For this review, take the finished solid that the model builds, in its own axes (mm). A direction names the side the tool comes from. Give positions to 0.01 mm unless a question says otherwise; leave off trailing zeros. Write each loop counter-clockwise with the first axis right and the second up, starting at its lowest first coordinate (ties: lowest second). Pieces come first, ordered by that corner, then holes. Notation, with made-up numbers: (86, 33) -> (143, 33) arc R17 ccw to (143, 42) -> close; hole circle Ø2 at (74.5, -11). An arc over 180 degrees is marked (long way). Return JSON: item names as keys, results as strings.
from build123d import *

# Parameters (mm, degrees)
SKETCH1_W           = 8
SKETCH1_H           = 1.2
SKETCH1_W_2         = 1
SKETCH1_H_2         = 4.1
REVOLVE1_ANGLE      = 180
SKETCH2_W           = 6.21
SKETCH2_H           = 1.5
CUT_EXTRUDE1_DEPTH  = 14.787313009
CUT_EXTRUDE2_DEPTH  = 14.787313009
SKETCH4_W           = 3.4
SKETCH4_H           = 2
BOSS_EXTRUDE1_DEPTH = 1.2
SKETCH6_W           = 2.8
SKETCH6_H           = 5
BOSS_EXTRUDE3_DEPTH = 1.2
BOSS_EXTRUDE4_DEPTH = 0.6
SKETCH8_W           = 4.65
SKETCH8_H           = 2.2
SKETCH8_W_2         = 16.704991512
SKETCH8_H_2         = 4.40240097
CUT_EXTRUDE3_DEPTH  = 10
SKETCH5_W           = 3.2
SKETCH5_H           = 5.3
BOSS_EXTRUDE5_DEPTH = 2.5
SKETCH9_W           = 2
SKETCH9_H           = 3.6
CUT_EXTRUDE4_DEPTH  = 5
CHAMFER1_SIZE       = 1


with BuildPart() as part:
    # Sketch1 → Revolve1 (revolve)
    with BuildSketch(Plane.XY):
        with Locations((4, 4.7)):
            Rectangle(SKETCH1_W, SKETCH1_H)
        with Locations((8.5, 4.7)):
            Rectangle(SKETCH1_W_2, SKETCH1_H)
        with Locations((8.5, 2.05)):
            Rectangle(SKETCH1_W_2, SKETCH1_H_2)
    revolve(axis=Axis((0, 0, 0), (0, 1, 0)), revolution_arc=REVOLVE1_ANGLE)

    # Sketch2 → Cut-Extrude1 (cut, through all)
    with BuildSketch(Plane.XY):
        with Locations((0, 3.35)):
            Rectangle(SKETCH2_W, SKETCH2_H)
    extrude(amount=-CUT_EXTRUDE1_DEPTH, mode=Mode.SUBTRACT)

    # Sketch3 → Cut-Extrude2 (cut, through all)
    with BuildSketch(Plane(origin=(0, 5.3, 0), x_dir=(1, 0, 0), z_dir=(0, 1, 0))):
        Polygon((-2.2, 5.8), (-3.6, 5.8), (-3.6, 0), (3.6, 0), (3.6, 5.8), (2.2, 5.8), (2.2, 0.8), (-2.2, 0.8), align=None)
    extrude(amount=-CUT_EXTRUDE2_DEPTH, mode=Mode.SUBTRACT)

    # Sketch4 → Boss-Extrude1 (add)
    with BuildSketch(Plane(origin=(0, 5.3, 0), x_dir=(1, 0, 0), z_dir=(0, 1, 0))):
        with Locations((5.3, -1)):
            Rectangle(SKETCH4_W, SKETCH4_H)
        with Locations((-5.3, -1)):
            Rectangle(SKETCH4_W, SKETCH4_H)
    extrude(amount=-BOSS_EXTRUDE1_DEPTH)

    # Sketch6 → Boss-Extrude3 (add)
    with BuildSketch(Plane.XY.offset(-0.8)):
        with Locations((0, 7.8)):
            Rectangle(SKETCH6_W, SKETCH6_H)
    extrude(amount=-BOSS_EXTRUDE3_DEPTH)

    # Sketch7 → Boss-Extrude4 (add, symmetric)
    with BuildSketch(Plane(origin=(0, 0, 0), x_dir=(0, 0, -1), z_dir=(1, 0, 0))):
        Polygon((2, 10.3), (9, 5.3), (2, 5.3), align=None)
    extrude(amount=BOSS_EXTRUDE4_DEPTH, both=True)

    # Sketch8 → Cut-Extrude3 (cut)
    with BuildSketch(Plane(origin=(0, 5.3, 0), x_dir=(1, 0, 0), z_dir=(0, 1, 0))):
        Polygon((-3.6, 0), (-3.6, 2.2), (-7.15, 2.2), (-7.15, 0), (-7, 0), align=None)
        with Locations((4.825, 1.1)):
            Rectangle(SKETCH8_W, SKETCH8_H)
        with Locations((1.202495756, -2.201200485)):
            Rectangle(SKETCH8_W_2, SKETCH8_H_2)
    extrude(amount=-CUT_EXTRUDE3_DEPTH, mode=Mode.SUBTRACT)

    # Sketch5 → Boss-Extrude5 (add)
    with BuildSketch(Plane(origin=(8, 0, 0), x_dir=(0, 0, -1), z_dir=(1, 0, 0))):
        with Locations((0, 2.65)):
            Rectangle(SKETCH5_W, SKETCH5_H)
    boss_extrude5 = extrude(amount=BOSS_EXTRUDE5_DEPTH)

    # Sketch9 → Cut-Extrude4 (cut)
    with BuildSketch(Plane(origin=(10.5, 0, 0), x_dir=(0, 0, -1), z_dir=(1, 0, 0))):
        with Locations((0.6, 2.65)):
            Rectangle(SKETCH9_W, SKETCH9_H)
    cut_extrude4 = extrude(amount=-CUT_EXTRUDE4_DEPTH, mode=Mode.SUBTRACT)

    # Mirror1: Boss-Extrude5, Cut-Extrude4 across plane
    add(boss_extrude5.mirror(Plane(origin=(0, 0, 0), x_dir=(0, 0, 1), z_dir=(1, 0, 0))))
    add(cut_extrude4.mirror(Plane(origin=(0, 0, 0), x_dir=(0, 0, 1), z_dir=(1, 0, 0))), mode=Mode.SUBTRACT)

    # Chamfer1
    chamfer1_edges = [part.edges().sort_by_distance(p)[0] for p in [
        (10.5, 4.875, -1.6),
        (10.5, 2.65, 1.6),
        (10.5, 0.425, -1.6),
        (-10.5, 2.65, 1.6),
        (-10.5, 4.875, -1.6),
        (-10.5, 0.425, -1.6),
    ]]
    chamfer(chamfer1_edges, length=CHAMFER1_SIZE)


solid = part.part
1. Add section A-A, the plane y = 2.25. State the section outline as (x, z) points, plus the area to 3 significant figures.
Results found:
{"outline": "(-10.5, 0.4) -> (-8, 0.4) -> (-8, 1.6) -> (-9.5, 1.6) -> (-10.5, 0.6) -> close; (-8.86, -1.6) arc R9 ccw to (8.86, -1.6) -> (7.84, -1.6) arc R8 cw to (-7.84, -1.6) -> close; (8, 0.4) -> (10.5, 0.4) -> (10.5, 0.6) -> (9.5, 1.6) -> (8, 1.6) -> close", "area": "28.5 mm²"}
2. The part is to be moulded in two halves that separate along Z. For faces 1 (the flat face through (9, 4.45, -1)), 2 (the flat face through (0, 10.3, -1)), 3 (the flat face through (-3, 5, -5.8)), say which applies: +Z half, -Z half, draft (parallel to the pull), parting line (faces both ways), or undercut.
Results found:
{"face 1": "undercut", "face 2": "draft", "face 3": "+Z half"}
3. For pin 1 (0.5 mm diameter, centred on x = -9.5, y = 0, fed in from -Z); pin 2 (1.5 mm diameter, centred on y = 7.5, z = -6, fed in from +X); pin 3 (0.7 mm diameter, centred on x = 7.5, y = 5, fed in from +Z), all flat-tipped, find the tip position at first contact; note any pin that passes through.
Results found:
{"pin 1": "stops at z = -1.6", "pin 2": "stops at x = 0.6", "pin 3": "stops at z = 0"}
4. Add section C-C, the plane y = 3.5. State the section outline as (x, z) points (3 decimals).
Results found:
{"outline": "(-10.5, 0.4) -> (-8, 0.4) -> (-8, 1.6) -> (-9.5, 1.6) -> (-10.5, 0.6) -> close; (-8.857, -1.6) arc R9 ccw to (-3.105, -8.447) -> (-3.105, -7.373) arc R8 cw to (-7.838, -1.6) -> close; (3.105, -8.447) arc R9 ccw to (8.857, -1.6) -> (7.838, -1.6) arc R8 cw to (3.105, -7.373) -> close; (8, 0.4) -> (10.5, 0.4) -> (10.5, 0.6) -> (9.5, 1.6) -> (8, 1.6) -> close"}
5. Add section B-B, the plane z = -3.25. State the section outline as (x, y) points, plus the area to 3 significant figures.
Results found:
{"outline": "(-8.39, 0) -> (-7.31, 0) -> (-7.31, 4.1) -> (-3.6, 4.1) -> (-3.6, 5.3) -> (-8.39, 5.3) -> close; (-2.2, 4.1) -> (2.2, 4.1) -> (2.2, 5.3) -> (0.6, 5.3) -> (0.6, 9.41) -> (-0.6, 9.41) -> (-0.6, 5.3) -> (-2.2, 5.3) -> close; (3.6, 4.1) -> (7.31, 4.1) -> (7.31, 0) -> (8.39, 0) -> (8.39, 5.3) -> (3.6, 5.3) -> close", "area": "30.6 mm²"}
6. For faces 4 (the cylindrical face through (0, 2, -8)), 5 (the flat face through (7.15, 5, -1)), 6 (the flat face through (9, 0.85, -1)), 7 (the flat face through (0.6, 7, -4)), list the 3-axis set-ups (+Z, -Z, +X, -X, +Y, -Y) from which the entire face can be reached by the end or side of a thin tool; tool diameter is ignored.
Results found:
{"face 4": "+Z, -Y", "face 5": "+Z, +Y, -Y", "face 6": "+X, -X", "face 7": "-Z, +X, +Y"}
7. To check wall thickness, follow probe 1 along Z at (x, y) = (8.25, 4); probe 2 along X at (y, z) = (4.5, -1); probe 3 along Y at (x, z) = (6.75, -5). State the ranges of each line that lie inside material, in increasing order.
Results found:
{"probe 1": "z = -3.6 to -1.6, 0.4 to 1.6", "probe 2": "x = -10.1 to -7.15, -2.2 to 2.2, 7.15 to 10.1", "probe 3": "y = 0 to 5.3"}
